from build123d import *

# Parameters (mm, degrees)
EXTRUDE_1_DEPTH      = 2
EXTRUDE_1_DEPTH_BACK = 2
SKETCH_1_W           = 4.5
SKETCH_1_H           = 4.5
SKETCH_2_W           = 2.5
SKETCH_2_H           = 2.5
CUT_EXTRUDE_1_DEPTH  = 1.5
FILLET_1_R           = 0.2


with BuildPart() as part:
    # Sketch 1 → Extrude 1 (new, two sides: drawn at the far end of the back side and taken through both)
    with BuildSketch(Plane(origin=(0, 0, 0), x_dir=(1, 0, 0), z_dir=(0, 1, 0)).offset(-EXTRUDE_1_DEPTH_BACK)):
        Rectangle(SKETCH_1_W, SKETCH_1_H)
    extrude(amount=EXTRUDE_1_DEPTH + EXTRUDE_1_DEPTH_BACK)

    # Sketch 2 → Cut-Extrude 1 (cut)
    with BuildSketch(Plane(origin=(0, 2, 0), x_dir=(1, 0, 0), z_dir=(0, 1, 0))):
        Rectangle(SKETCH_2_W, SKETCH_2_H)
    cut_extrude_1 = extrude(amount=-CUT_EXTRUDE_1_DEPTH, mode=Mode.SUBTRACT)

    # Mirror 1: Cut-Extrude 1 across plane
    add(cut_extrude_1.mirror(Plane.ZX), mode=Mode.SUBTRACT)

    # Sketch 3 → Revolve 1 (revolve)
    with BuildSketch(Plane(origin=(0, 0, 0), x_dir=(1, 0, 0), z_dir=(0, 1, 0)), mode=Mode.PRIVATE) as revolve_1_sk:
        with BuildLine():
            Line((0, 2.25), (-0.7, 2.25))
            Line((-0.7, 2.25), (-0.7, 2.95))
            ThreePointArc((-0.7, 2.95), (-0.494974747, 3.444974747), (0, 3.65))
            Line((0, 3.65), (0, 2.95))
            Line((0, 2.95), (0, 2.25))
        make_face()
    revolve_1 = revolve(revolve_1_sk.sketch.rotate(Axis((0, 0, -2.95), (0, 0, -1)), 180), axis=Axis((0, 0, -2.95), (0, 0, -1)))

    # Mirror 2: Revolve 1 across plane
    add(revolve_1.mirror(Plane.XY))

    # Sketch 5 → Revolve 2 (revolve)
    with BuildSketch(Plane(origin=(0, 0, 0), x_dir=(1, 0, 0), z_dir=(0, 1, 0))):
        with BuildLine():
            Line((-2.25, 0), (-2.95, 0))
            Line((-2.95, 0), (-3.65, 0))
            ThreePointArc((-3.65, 0), (-3.444974747, 0.494974747), (-2.95, 0.7))
            Line((-2.95, 0.7), (-2.25, 0.7))
            Line((-2.25, 0.7), (-2.25, 0))
        make_face()
    revolve_2 = revolve(axis=Axis((-2.25, 0, 0), (-1, 0, 0)))

    # Mirror 3: Revolve 2 across plane
    add(revolve_2.mirror(Plane(origin=(0, 0, 0), x_dir=(0, 0, 1), z_dir=(1, 0, 0))))

    # Fillet 1
    fillet_1_edges = [part.edges().sort_by_distance(p)[0] for p in [
        (0, -2, 2.25),
        (0, 2, -2.25),
        (-2.25, 2, 0),
        (2.25, -2, 0),
        (0, 2, 2.25),
        (2.25, 2, 0),
        (0, 2, -1.25),
        (-1.25, 2, 0),
        (0, 2, 1.25),
        (1.25, 2, 0),
        (0, -2, -1.25),
        (-1.25, -2, 0),
        (0, -2, 1.25),
        (1.25, -2, 0),
        (0, -2, -2.25),
        (-2.25, -2, 0),
        (2.25, 0, -2.25),
        (2.25, 0, 2.25),
        (-2.25, 0, 2.25),
        (-2.25, 0, -2.25),
    ]]
    fillet(fillet_1_edges, radius=FILLET_1_R)


solid = part.part
Geometry: final body of the model. Coordinates: model frame, mm. A direction names the side the tool comes from. Give positions to 0.01 mm unless a question says otherwise; leave off trailing zeros. Write each loop counter-clockwise with the first axis right and the second up, starting at its lowest first coordinate (ties: lowest second). Pieces come first, ordered by that corner, then holes. Notation, with made-up numbers: (39, 67) -> (62, 67) arc R13 cw to (62, 87) -> close; hole circle Ø8 at (45.5, -18.75). An arc over 180 degrees is marked (long way). Answer as a JSON object with one key per item and string values.
1. Cut plane A-A on y = -0.9. Output: boundary loops of the cut face in (x, z).
Ans:
{"outline": "(-2.25, -2.05) arc R0.2 ccw to (-2.05, -2.25) -> (2.05, -2.25) arc R0.2 ccw to (2.25, -2.05) -> (2.25, 2.05) arc R0.2 ccw to (2.05, 2.25) -> (-2.05, 2.25) arc R0.2 ccw to (-2.25, 2.05) -> close; hole (-1.25, -1.25) -> (1.25, -1.25) -> (1.25, 1.25) -> (-1.25, 1.25) -> close"}
2. Contact query for flat-ended pins moving along their axis: pin 1 (1.4 mm diameter, centred on x = 0.5, y = -1, fed in from -Z); pin 2 (1 mm diameter, centred on x = 0.5, y = 0.5, fed in from -Z); pin 3 (1 mm diameter, centred on y = -1, z = 0, fed in from +X); pin 4 (1.1 mm diameter, centred on y = 0, z = -0.5, fed in from +X). Output: stop coordinate, or through.
Ans:
{"pin 1": "stops at z = -3.51", "pin 2": "stops at z = -3.62", "pin 3": "stops at x = 3.44", "pin 4": "stops at x = 3.65"}
3. Cut plane C-C on y = 0. Output: boundary loops of the cut face in (x, z), and give its area (3 significant figures).
Ans:
{"outline": "(-2.95, -0.7) -> (-2.25, -0.7) -> (-2.25, -2.05) arc R0.2 ccw to (-2.05, -2.25) -> (-0.7, -2.25) -> (-0.7, -2.95) arc R0.7 ccw to (0.7, -2.95) -> (0.7, -2.25) -> (2.05, -2.25) arc R0.2 ccw to (2.25, -2.05) -> (2.25, -0.7) -> (2.95, -0.7) arc R0.7 ccw to (2.95, 0.7) -> (2.25, 0.7) -> (2.25, 2.05) arc R0.2 ccw to (2.05, 2.25) -> (0.7, 2.25) -> (0.7, 2.95) arc R0.7 ccw to (-0.7, 2.95) -> (-0.7, 2.25) -> (-2.05, 2.25) arc R0.2 ccw to (-2.25, 2.05) -> (-2.25, 0.7) -> (-2.95, 0.7) arc R0.7 ccw to start", "area": "27.2 mm^2"}
4. Cut plane B-B on x = 0. Output: boundary loops of the cut face in (y, z), and give its area (3 significant figures).
Ans:
{"outline": "(-2, -2.05) arc R0.2 ccw to (-1.8, -2.25) -> (-0.7, -2.25) -> (-0.7, -2.95) arc R0.7 ccw to (0.7, -2.95) -> (0.7, -2.25) -> (1.8, -2.25) arc R0.2 ccw to (2, -2.05) -> (2, -1.45) arc R0.2 ccw to (1.8, -1.25) -> (0.5, -1.25) -> (0.5, 1.25) -> (1.8, 1.25) arc R0.2 ccw to (2, 1.45) -> (2, 2.05) arc R0.2 ccw to (1.8, 2.25) -> (0.7, 2.25) -> (0.7, 2.95) arc R0.7 ccw to (-0.7, 2.95) -> (-0.7, 2.25) -> (-1.8, 2.25) arc R0.2 ccw to (-2, 2.05) -> (-2, 1.45) arc R0.2 ccw to (-1.8, 1.25) -> (-0.5, 1.25) -> (-0.5, -1.25) -> (-1.8, -1.25) arc R0.2 ccw to (-2, -1.45) -> close", "area": "13.9 mm^2"}
5. Access query for faces 5 (the flat face through (-1.25, -1, 0)), 6 (the flat face through (2.25, -1, 0)), 7 (the flat face through (-1.25, 1, 0)). Directions: +Z, -Z, +X, -X, +Y, -Y. A direction counts if a zero-diameter tool reaches every point of the face in a straight line with its end or side. Return the directions, or none.
Ans:
{"face 5": "-Y", "face 6": "+X", "face 7": "+Y"}
6. Cut plane D-D on z = 1. Output: boundary loops of the cut face in (x, y).
Ans:
{"outline": "(-2.25, -1.8) arc R0.2 ccw to (-2.05, -2) -> (-1.45, -2) arc R0.2 ccw to (-1.25, -1.8) -> (-1.25, -0.5) -> (1.25, -0.5) -> (1.25, -1.8) arc R0.2 ccw to (1.45, -2) -> (2.05, -2) arc R0.2 ccw to (2.25, -1.8) -> (2.25, 1.8) arc R0.2 ccw to (2.05, 2) -> (1.45, 2) arc R0.2 ccw to (1.25, 1.8) -> (1.25, 0.5) -> (-1.25, 0.5) -> (-1.25, 1.8) arc R0.2 ccw to (-1.45, 2) -> (-2.05, 2) arc R0.2 ccw to (-2.25, 1.8) -> close"}
7. Mould query, pull axis Z, two halves, no side actions, for faces 1 (the flat face through (0, -1, -2.25)), 2 (the flat face through (0, 1, -1.25)), 3 (the cylindrical face through (-2.6, 0, 0.7)), 4 (the flat face through (-1.85, -2, -0.03)). Classes: pulls with the +Z half, pulls with the -Z half, needs draft (parallel to the pull), parting line crosses it, or undercut.
Ans:
{"face 1": "pulls with the -Z half", "face 2": "undercut", "face 3": "parting line crosses it", "face 4": "needs draft"}
8. Ray query, probe 1 along Z at (x, y) = (-1, -0.8); probe 2 along Z at (x, y) = (1.5, -0.55). Return the intervals inside material, ascending. Write a range as from..to.
Ans:
{"probe 1": "z = -2.25..-1.25, 1.25..2.25", "probe 2": "z = -2.25..2.25"}
